Geometry check sheet. Reference: the model listing, model coordinates, mm. A direction names the side the tool comes from. Round coordinates to 2 decimals unless told otherwise and drop trailing zeros. Write each loop counter-clockwise with the first axis right and the second up, starting at its lowest first coordinate (ties: lowest second). Pieces come first, ordered by that corner, then holes.
from build123d import *

# Parameters (mm, degrees)
REVOLVE1_ANGLE                  = 180
BOSS_EXTRUDE1_START             = -11
BOSS_EXTRUDE1_DEPTH             = 11
CUT_EXTRUDE1_REACH              = 68.374
BOSS_EXTRUDE2_REACH             = 67.327
BOSS_EXTRUDE2_END_RADIUS        = 40.5
SKETCH6_W                       = 25.4
SKETCH6_H                       = 18
BOSS_EXTRUDE2_DIRECTION_2_DEPTH = 15
SKETCH8_W                       = 4
SKETCH8_H                       = 19.884534
CUT_EXTRUDE3_DEPTH              = 80.722348
FILLET1_START                   = 2
FILLET1_DEPTH                   = 5
FILLET1_START_2                 = -11
FILLET1_2_DEPTH                 = 16.09884
FILLET1_START_3                 = 37
FILLET1_3_DEPTH                 = 28
FILLET1_START_4                 = 62
FILLET1_4_OUTLINE_W             = 4
FILLET1_4_OUTLINE_H             = 5
FILLET1_4_DEPTH                 = 3
FILLET1_START_5                 = 39.17071
FILLET1_5_OUTLINE_W             = 4
FILLET1_5_OUTLINE_H             = 5
FILLET1_5_DEPTH                 = 2.944756
FILLET1_6_DEPTH                 = 6
SKETCH9_R                       = 2
BOSS_EXTRUDE3_DEPTH             = 10
CUT_EXTRUDE4_DEPTH              = 75.187772
CUT_EXTRUDE4_DEPTH_BACK         = 5
CUT_EXTRUDE5_DEPTH              = 85.064413
SKETCH12_W                      = 14.911662
SKETCH12_H                      = 13.358131
SKETCH12_W_2                    = 10
SKETCH12_H_2                    = 8
BOSS_EXTRUDE4_DEPTH             = 15
FILLET2_R                       = 5


with BuildPart() as part:
    # Sketch2 → Revolve1 (revolve, symmetric)
    with BuildSketch(Plane(origin=(0, 0, 0), x_dir=(0, 0, -1), z_dir=(1, 0, 0))) as revolve1_sk:
        Polygon((-34, -11), (-35.5, -9.5), (-35.5, 9.5), (-34, 11), (-35.5, 11), (-40.5, 11), (-40.5, -11), (-35.5, -11), align=None)
    revolve(axis=Axis((0, 0, 0), (0, 1, 0)), revolution_arc=REVOLVE1_ANGLE / 2)
    revolve(revolve1_sk.sketch, axis=Axis((0, 0, 0), (0, -1, 0)), revolution_arc=REVOLVE1_ANGLE / 2)

    # Sketch3 → Boss-Extrude1 (add)
    with BuildSketch(Plane(origin=(0, 0, 0), x_dir=(1, 0, 0), z_dir=(0, 1, 0)).offset(BOSS_EXTRUDE1_START)):
        with BuildLine():
            ThreePointArc((-40.5, 0), (0, -40.5), (40.5, 0))
            add(Edge.make_bspline(
                [(40.5, 0), (41.574904, -20.679763), (31.861074, -51.110818), (0, -51.360442)],
                knots=[0, 0, 0, 0, 1, 1, 1, 1], degree=3))
            add(Edge.make_bspline(
                [(-40.5, 0), (-41.574904, -20.679763), (-31.861074, -51.110818), (0, -51.360442)],
                knots=[0, 0, 0, 0, 1, 1, 1, 1], degree=3))
        make_face()
    extrude(amount=BOSS_EXTRUDE1_DEPTH)

    # Sketch5 → Cut-Extrude1 (cut, up to next)
    with BuildSketch(Plane(origin=(0, 0, 0), x_dir=(1, 0, 0), z_dir=(0, 1, 0)), mode=Mode.PRIVATE) as cut_extrude1_sk1:
        Polygon((32.298595, -50), (-32.298595, -50), (-4.520904, -70.798059), align=None)
    cut_extrude1_tool1 = extrude(cut_extrude1_sk1.sketch, amount=-CUT_EXTRUDE1_REACH, mode=Mode.PRIVATE) & part.part
    add(cut_extrude1_tool1.solids().sort_by_distance((-1.506968, 0, 56.932686))[0], mode=Mode.SUBTRACT)

    # Boss-Extrude2: up to this cylinder (the profile starts outside it)
    boss_extrude2_end = Plane(origin=(0, -2, 0), z_dir=(0, -1, 0)) * Cylinder(BOSS_EXTRUDE2_END_RADIUS, 216.654, mode=Mode.PRIVATE)
    # Sketch6 → Boss-Extrude2 (add, up to the surface)
    with BuildSketch(Plane.XY.offset(50), mode=Mode.PRIVATE) as boss_extrude2_sk1:
        with Locations((0, -2)):
            Rectangle(SKETCH6_W, SKETCH6_H)
    boss_extrude2_tool1 = extrude(boss_extrude2_sk1.sketch, amount=-BOSS_EXTRUDE2_REACH, mode=Mode.PRIVATE) - boss_extrude2_end
    add(boss_extrude2_tool1.solids().sort_by_distance((0, -2, 50))[0])

    # Sketch6 → Boss-Extrude2 direction 2 (add)
    with BuildSketch(Plane.XY.offset(50)):
        with Locations((0, -2)):
            Rectangle(SKETCH6_W, SKETCH6_H)
    extrude(amount=BOSS_EXTRUDE2_DIRECTION_2_DEPTH)

    # Sketch8 → Cut-Extrude3 (cut, through all)
    with BuildSketch(Plane(origin=(0, 11, 0), x_dir=(1, 0, 0), z_dir=(0, 1, 0))):
        with BuildLine():
            Line((15.113165, -40.129156), (15.113165, -45.006528))
            add(Edge.make_bspline(
                [(15.113165, -45.006528), (20.553217, -43.096096), (30.745136, -32.716473), (33.442003, -26.840069)],
                knots=[0, 0, 0, 0, 1, 1, 1, 1], degree=3))
            ThreePointArc((33.442003, -26.840069), (25.17044, -34.716075), (15.113165, -40.129156))
        make_face()
        with BuildLine():
            Line((-15.113165, -40.129156), (-15.113165, -45.006528))
            add(Edge.make_bspline(
                [(-15.113165, -45.006528), (-20.553217, -43.096096), (-30.745136, -32.716473), (-33.442003, -26.840069)],
                knots=[0, 0, 0, 0, 1, 1, 1, 1], degree=3))
            ThreePointArc((-33.442003, -26.840069), (-25.17044, -34.716075), (-15.113165, -40.129156))
        make_face()
        with Locations((0, -52.057733)):
            Rectangle(SKETCH8_W, SKETCH8_H)
    extrude(amount=-CUT_EXTRUDE3_DEPTH, mode=Mode.SUBTRACT)

    # Fillet1: read off the stored shape, not the designer's step
    # Fillet1 outline → Fillet1 (cut)
    with BuildSketch(Plane(origin=(0, 0, 0), x_dir=(1, 0, 0), z_dir=(0, 1, 0)).offset(FILLET1_START)):
        with BuildLine():
            Line((-12.7, -65), (12.7, -65))
            Line((12.7, -65), (12.7, -38.457249))
            ThreePointArc((12.7, -38.457249), (0, -40.5), (-12.7, -38.457249))
            Line((-12.7, -38.457249), (-12.7, -65))
        make_face()
    extrude(amount=FILLET1_DEPTH, mode=Mode.SUBTRACT)

    # Fillet1 2 outline → Fillet1 2 (cut)
    with BuildSketch(Plane(origin=(0, 0, 0), x_dir=(1, 0, 0), z_dir=(0, 1, 0)).offset(FILLET1_START_2)):
        with BuildLine():
            Line((-12.7, -65), (-7.7, -65))
            add(Edge.make_bspline(
                [(-7.7, -65), (-12.7, -65), (-12.7, -60)],
                knots=[0, 0, 0, 1, 1, 1], degree=2, weights=[1, 0.707107, 1]))
            Line((-12.7, -60), (-12.7, -65))
        make_face()
        with BuildLine():
            add(Edge.make_bspline(
                [(7.7, -65), (12.7, -65), (12.7, -60)],
                knots=[0, 0, 0, 1, 1, 1], degree=2, weights=[1, 0.707107, 1]))
            Line((7.7, -65), (12.7, -65))
            Line((12.7, -65), (12.7, -60))
        make_face()
    extrude(amount=FILLET1_2_DEPTH, mode=Mode.SUBTRACT)

    # Fillet1 3 outline → Fillet1 3 (add)
    with BuildSketch(Plane.XY.offset(FILLET1_START_3)):
        with BuildLine():
            add(Edge.make_bspline(
                [(-12.7, 2), (-12.7, 7), (-7.7, 7)],
                knots=[0, 0, 0, 1, 1, 1], degree=2, weights=[1, 0.707107, 1]))
            Line((-12.7, 2), (-2, 2))
            Line((-2, 2), (-2, 7))
            Line((-2, 7), (-7.7, 7))
        make_face()
        with BuildLine():
            Line((2, 7), (2, 2))
            Line((2, 2), (12.7, 2))
            add(Edge.make_bspline(
                [(7.7, 7), (12.7, 7), (12.7, 2)],
                knots=[0, 0, 0, 1, 1, 1], degree=2, weights=[1, 0.707107, 1]))
            Line((7.7, 7), (2, 7))
        make_face()
    extrude(amount=FILLET1_3_DEPTH)

    # Fillet1 4 outline → Fillet1 4 (add)
    with BuildSketch(Plane.XY.offset(FILLET1_START_4)):
        with Locations((0, 4.5)):
            Rectangle(FILLET1_4_OUTLINE_W, FILLET1_4_OUTLINE_H)
    extrude(amount=FILLET1_4_DEPTH)

    # Fillet1 5 outline → Fillet1 5 (add)
    with BuildSketch(Plane.XY.offset(FILLET1_START_5)):
        with Locations((0, 4.5)):
            Rectangle(FILLET1_5_OUTLINE_W, FILLET1_5_OUTLINE_H)
    extrude(amount=FILLET1_5_DEPTH)

    # Fillet1 6 outline → Fillet1 6 (cut)
    with BuildSketch(Plane(origin=(0, 0, 0), x_dir=(1, 0, 0), z_dir=(0, 1, 0)).offset(FILLET1_START)):
        with BuildLine():
            Line((-12.7, -65), (-7.7, -65))
            add(Edge.make_bspline(
                [(-12.7, -60), (-12.7, -60.274102), (-12.679965, -60.548369), (-12.639842, -60.820553), (-12.536378, -61.284433), (-12.482162, -61.478121), (-12.41762, -61.668662), (-12.288664, -61.991396), (-12.22893, -62.125441), (-12.163988, -62.25706), (-11.922281, -62.702191), (-11.720174, -63.002028), (-11.490067, -63.281001), (-10.981001, -63.790067), (-10.702028, -64.020174), (-10.402191, -64.222281), (-9.95706, -64.463988), (-9.825441, -64.52893), (-9.691396, -64.588664), (-9.368662, -64.71762), (-9.178121, -64.782162), (-8.984433, -64.836378), (-8.520553, -64.939842), (-8.248369, -64.979965), (-7.974102, -65), (-7.7, -65)],
                knots=[0, 0, 0, 0, 0, 0.139857, 0.139857, 0.139857, 0.242164, 0.242164, 0.242164, 0.316823, 0.316823, 0.316823, 0.5, 0.5, 0.5, 0.683177, 0.683177, 0.683177, 0.757836, 0.757836, 0.757836, 0.860143, 0.860143, 0.860143, 1, 1, 1, 1, 1], degree=4))
            Line((-12.7, -60), (-12.7, -65))
        make_face()
        with BuildLine():
            Line((12.7, -65), (12.7, -60))
            add(Edge.make_bspline(
                [(12.7, -60), (12.7, -60.274102), (12.679965, -60.548369), (12.639842, -60.820553), (12.536378, -61.284433), (12.482162, -61.478121), (12.41762, -61.668662), (12.288664, -61.991396), (12.22893, -62.125441), (12.163988, -62.25706), (11.922281, -62.702191), (11.720174, -63.002028), (11.490067, -63.281001), (10.981001, -63.790067), (10.702028, -64.020174), (10.402191, -64.222281), (9.95706, -64.463988), (9.825441, -64.52893), (9.691396, -64.588664), (9.368662, -64.71762), (9.178121, -64.782162), (8.984433, -64.836378), (8.520553, -64.939842), (8.248369, -64.979965), (7.974102, -65), (7.7, -65)],
                knots=[0, 0, 0, 0, 0, 0.139857, 0.139857, 0.139857, 0.242164, 0.242164, 0.242164, 0.316823, 0.316823, 0.316823, 0.5, 0.5, 0.5, 0.683177, 0.683177, 0.683177, 0.757836, 0.757836, 0.757836, 0.860143, 0.860143, 0.860143, 1, 1, 1, 1, 1], degree=4))
            Line((7.7, -65), (12.7, -65))
        make_face()
    extrude(amount=FILLET1_6_DEPTH, mode=Mode.SUBTRACT)

    # Sketch9 → Boss-Extrude3 (add)
    # profile 1 of 2: a face of its own
    with BuildSketch(Plane.XY):
        with BuildLine():
            ThreePointArc((39.222943, -0.011905), (42.578982, -10.999961), (45.856052, 0.011905))
            ThreePointArc((45.856052, 0.011905), (42.500013, 10.999961), (39.222943, -0.011905))
        make_face()
        with Locations((42.557445, -5)):
            Circle(SKETCH9_R, mode=Mode.SUBTRACT)
        with Locations((42.52155, 5)):
            Circle(SKETCH9_R, mode=Mode.SUBTRACT)
    # profile 2 of 2: a face of its own
    with BuildSketch(Plane.XY):
        with BuildLine():
            ThreePointArc((-39.222943, -0.011905), (-42.578982, -10.999961), (-45.856052, 0.011905))
            ThreePointArc((-45.856052, 0.011905), (-42.500013, 10.999961), (-39.222943, -0.011905))
        make_face()
        with Locations(Location((-42.557445, -5, 0), (0, 0, 180))):
            Circle(SKETCH9_R, mode=Mode.SUBTRACT)
        with Locations(Location((-42.52155, 5, 0), (0, 0, 180))):
            Circle(SKETCH9_R, mode=Mode.SUBTRACT)
    extrude(amount=BOSS_EXTRUDE3_DEPTH)

    # Sketch10 → Cut-Extrude4 (cut, two sides: drawn at the far end of the back side and taken through both)
    with BuildSketch(Plane.XY.offset(10).offset(-CUT_EXTRUDE4_DEPTH_BACK)):
        with BuildLine():
            Line((39.407769, -9.137577), (39.407769, 9.164657))
            ThreePointArc((39.407769, 9.164657), (47.176604, 7.317427), (43.967661, 0.005126))
            ThreePointArc((43.967661, 0.005126), (47.210797, -7.320844), (39.407769, -9.137577))
        make_face()
        with BuildLine():
            Line((-39.407769, -9.137577), (-39.407769, 9.164657))
            ThreePointArc((-39.407769, 9.164657), (-47.176604, 7.317427), (-43.967661, 0.005126))
            ThreePointArc((-43.967661, 0.005126), (-47.210797, -7.320844), (-39.407769, -9.137577))
        make_face()
    extrude(amount=CUT_EXTRUDE4_DEPTH + CUT_EXTRUDE4_DEPTH_BACK, mode=Mode.SUBTRACT)

    # Sketch11 → Cut-Extrude5 (cut, through all)
    with BuildSketch(Plane(origin=(0, 11, 0), x_dir=(1, 0, 0), z_dir=(0, 1, 0))):
        with BuildLine():
            Line((48.52155, -10), (39.246019, -10))
            ThreePointArc((39.246019, -10), (0, -40.5), (-39.246019, -10))
            Line((-39.246019, -10), (-48.52155, -10))
            Line((-48.52155, -10), (-48.52155, -69.748878))
            Line((-48.52155, -69.748878), (48.52155, -69.748878))
            Line((48.52155, -69.748878), (48.52155, -10))
        make_face()
    extrude(amount=-CUT_EXTRUDE5_DEPTH, mode=Mode.SUBTRACT)

    # Sketch12 → Boss-Extrude4 (add)
    with BuildSketch(Plane(origin=(0, 11, 0), x_dir=(1, 0, 0), z_dir=(0, 1, 0))):
        with Locations((0, -44.956584)):
            Rectangle(SKETCH12_W, SKETCH12_H)
        with Locations((0, -44.956584)):
            Rectangle(SKETCH12_W_2, SKETCH12_H_2, mode=Mode.SUBTRACT)
    extrude(amount=-BOSS_EXTRUDE4_DEPTH)

    # Fillet2
    fillet2_edges = [part.edges().sort_by_distance(p)[0] for p in [
        (-7.455831, 3.5, 51.635649),
        (7.455831, 3.5, 51.635649),
    ]]
    fillet(fillet2_edges, radius=FILLET2_R)


solid = part.part
1. Depth check by flat-ended pin: pin 1 Ø6 at (y, z) = (2.5, 36) entering from -X; pin 2 Ø4 at (x, y) = (10, 5.5) entering from +Z; pin 3 Ø12 at (x, y) = (-42.52, 5) entering from -Z; pin 4 Ø3 at (x, y) = (43, -1.5) entering from +Z. Enter the tip coordinate at first touch or a pass-through.
2. Access from +Z, -Z, +X, -X, +Y, -Y to the whole of each face (thin tool, end or side, straight path). Record for faces 4 (the face through (0.75, 10.76, 34.23)), 5 (the face through (-43.6, 0.1, 5)), 6 (the face through (-45.6, 0.1, 10)), 7 (the face through (0, 4, 40.957)).
3. Section check C-C (x = -38). Record the cut outline in (y, z), plus the area to 3 significant figures.
4. Scan lines: line 1 along X through (y, z) = (-5, 1.7); line 2 along X through (y, z) = (-5, 8.1); line 3 along Z through (x, y) = (-4, 7). Record each from-to range of solid material in increasing order.
5. Section check B-B (y = 1). Record the cut outline in (x, z), plus the area to 3 significant figures.
6. Release check for a two-part mould opening along Y. For faces 1 (the face through (-7.456, 4, 43)), 2 (the face through (44.43, 5.6, 2.46)), 3 (the face through (0, -11, 35)) record: +Y half, -Y half, draft (parallel to the pull), parting line (faces both ways), or undercut.
7. Section check A-A (x = 0). Record the cut outline in (y, z), plus the area to 3 significant figures.
Results below:
1. pin 1: stops at x = -23.48
1. pin 2: stops at z = 39.7
1. pin 3: stops at z = 0
1. pin 4: stops at z = 5
2. face 4: -Z
2. face 5: +Z
2. face 6: +Z, -X, +Y, -Y
2. face 7: +Y, -Y
3. outline: (-11, 0) - (11, 0) - (11, 14.01) - (-11, 14.01) - close
3. area: 308 mm2
4. line 1: x = -48.56 to -44.56, -40.56 to -35.46, 35.46 to 40.56, 44.56 to 48.56
4. line 2: x = -48.56 to -47.76, -39.41 to -34.56, 34.56 to 39.41, 47.76 to 48.56
4. line 3: z = 35.27 to 40.96, 48.96 to 51.39
5. outline: (-46.99, 0) - (-35.5, 0) arc R35.5 cw to (35.5, 0) - (46.99, 0) - (46.99, 10) - (45.84, 10) - (45.84, 5) - (39.41, 5) - (39.41, 10) - (39.25, 10) arc R40.5 ccw to (7.46, 39.81) - (7.46, 46.64) arc R5 ccw to (2.46, 51.64) - (-2.46, 51.64) arc R5 ccw to (-7.46, 46.64) - (-7.46, 39.81) arc R40.5 ccw to (-39.25, 10) - (-39.41, 10) - (-39.41, 5) - (-45.84, 5) - (-45.84, 10) - (-46.99, 10) - close; hole (-5, 40.96) - (5, 40.96) - (5, 48.96) - (-5, 48.96) - close
5. area: 749 mm2
6. face 1: draft
6. face 2: undercut
6. face 3: -Y half
7. outline: (-11, 34) - (-9.5, 35.5) - (9.5, 35.5) - (11, 34) - (11, 40.96) - (-4, 40.96) - (-4, 40.5) - (-11, 40.5) - close; (-4, 48.96) - (11, 48.96) - (11, 51.64) - (-4, 51.64) - close
7. area: 159 mm2
